Autodesk Fusion 360 part; units mm, degrees
ref_plane "WorkPlane1" through (4, 0, 0) normal (1, 0, 0) x (0, 1, 0)
sketch "Sketch2" plane through (0, 0, 0) normal (1, 0, 0) x (0, 1, 0)
  line L0 (-12, 0) -> (-16, 0)
  line L1 (-16, 0) -> (-16, 5)
  line L2 (-16, 5) -> (-12, 5)
  line L3 (-12, 5) -> (-12, 0)
  line L4 (12, 0) -> (16, 0)
  line L5 (16, 0) -> (16, 5)
  line L6 (16, 5) -> (12, 5)
  line L7 (12, 5) -> (12, 0)
  line L8 (-12, 5) -> (12, 5)
  line L9 (12, 5) -> (12, 0)
  line L10 (12, 0) -> (-12, 0)
  line L11 (-12, 0) -> (-12, 5)
extrude "Extrude1" add sketch "Sketch2" along normal blind 7 contours L3 L7 L8 L9 L10 L11 makes body 1
extrude "Extrude2" add sketch "Sketch2" along normal blind 44 separate body contours L0 L1 L2 L3 L11 | L4 L5 L6 L7 L9 makes body 2 at (29.3333, -16, 1.6667) makes body 3 at (29.3333, 12, 3.3333)
fillet "Fillet1" radius 5 2 edges at (44, -14, 5) (44, 14, 5) on bodies 2 3
sketch "Sketch3" plane through (0, 0, 0) normal (0, 1, 0) x (1, 0, 0)
  circle A0 centre (39, 0) radius 1
  dimension "d8" = 2
sketch "Sketch4" plane through (0, 0, 0) normal (1, 0, 0) x (0, 1, 0)
  circle A0 centre (0, 0) radius 5
extrude "Extrude4" add sketch "Sketch4" against normal blind 33 bodies 1
shell "Shell1" thickness 2 removed faces 1 at (-33, -1.5016, -0.7231) on bodies 1
ref_plane "WorkPlane2" through (-2, 0, 0) normal (1, 0, 0) x (0, 1, 0)
sketch "Sketch7" plane through (-2, 0, 0) normal (1, 0, 0) x (0, 1, 0)
sketch "Sketch8" plane through (0, 0, 0) normal (1, 0, 0) x (0, 1, 0)
  circle A0 centre (0, 0) radius 3
extrude "Extrude6" add sketch "Sketch8" against normal blind 29 bodies 1
extrude "Extrude8" add 5 faces at (4.6667, 1.6667, 0) (14.6667, -13.3333, 0) (14.6667, 13.3333, 0) (14.6667, 13.3333, 0) (14.6667, -13.3333, 0) along direction (0, 0, -1) blind 5 on bodies 1 2 3 bodies 1 2 3
fillet "Fillet2" radius 5 2 edges at (44, 14, -5) (44, -14, -5) on bodies 1
extrude "Extrude12" cut sketch "Sketch3" along normal mid plane 48 bodies 1 1
fillet "Fillet3" radius 3 2 edges at (0, -16, 0) (0, 16, 0) on bodies 1
fillet "Fillet4" radius 3 2 edges at (7, -12, 0) (7, 12, 0) on bodies 1
Could you check a few things on this model? Use its own coordinates, in mm. A direction names the side the tool comes from. Give positions to 0.01 mm unless a question says otherwise; leave off trailing zeros. Write each loop counter-clockwise with the first axis right and the second up, starting at its lowest first coordinate (ties: lowest second). Pieces come first, ordered by that corner, then holes. Notation, with made-up numbers: (-13, -22) - (20, -22) arc R16 ccw to (20, -18) - close; hole circle Ø3 at (14, -30.75). An arc over 180 degrees is marked (long way). Use CSV: the item, a comma, the result in double quotes. Start each with the question number.
Item 1: I want a section at B-B, the plane x = -26. Please give me the cut outline in (y, z).
Item 2: If I drill on line 1 along Y through (x, z) = (14, 3.5); line 2 along X through (y, z) = (-13.2, 0); line 3 along Z through (x, y) = (39, -13.7), over which ranges is the centre line in solid material (lowest first)?
Item 3: For faces 1 (the face through (43, 14, -3)), 2 (the face through (7.9, 11.14, 0.07)), 3 (the face through (3, 0, 2)), 4 (the face through (-31, -3, 0)), which set-ups out of +Z, -Z, +X, -X, +Y, -Y let a thin tool reach every point of the face, with its end or its side?
Item 4: I'm going to push flat-ended pins straight in: pin 1 (5 mm diameter, centred on y = 9.5, z = -0.5, fed in from -X); pin 2 (1.1 mm diameter, centred on y = 0.5, z = 2.5, fed in from +X); pin 3 (1 mm diameter, centred on x = 1, z = -3, fed in from +Y). Where does each tip first touch, or does it pass through?
Item 5: I want a section at A-A, the plane x = 25.5. Please give me the cut outline in (y, z).
Item 6: If we mould it in two halves opening along X, with no side actions, what happens to faces 5 (the face through (23, -16, 0)), 6 (the face through (4, 0, 3)), 7 (the face through (42, -14, 4))? For each: pulls with the +X half, pulls with the -X half, needs draft (parallel to the pull), parting line crosses it, or undercut.
Findings:
1,outline,"circle Ø10 at (0, 0)"
2,line 1,"y = -16 to -12, 12 to 16"
2,line 2,"x = 0.01 to 38, 40 to 44"
2,line 3,"z = -5 to -1, 1 to 5"
3,face 1,"-Z, +X, +Y, -Y"
3,face 2,"+Z, -Z, +X"
3,face 3,"none"
3,face 4,"-X"
4,pin 1,"stops at x = 0"
4,pin 2,"stops at x = 7"
4,pin 3,"stops at y = 15.6"
5,outline,"(-16, -5) - (-12, -5) - (-12, 5) - (-16, 5) - close; (12, -5) - (16, -5) - (16, 5) - (12, 5) - close"
6,face 5,"needs draft"
6,face 6,"undercut"
6,face 7,"pulls with the +X half"
